Here's how the part is built. I have some questions about the finished solid (model axes, mm). Give positions to 0.01 mm unless a question says otherwise; leave off trailing zeros. Loops run counter-clockwise (first coordinate to the right, second up) from the corner with the lowest first, then second, coordinate; pieces in that order, holes last.
Q1. I'm going to push flat-ended pins straight in: P1, Ø4, axis at y = 23.5, z = 4, coming from the -X side; P2, Ø2.5, axis at y = 22.5, z = 3.5, coming from the +X side; P3, Ø5, axis at x = 93, y = -5, coming from the -Z side; P4, Ø4, axis at x = -65.5, z = 5.5, coming from the +Y side. Where does each tip first touch, or does it pass through?
Q2. Suppose I cut it at A-A (y = -19.5). List the corners of the cut face in (x, z) for me.
Q3. I need wall thicknesses on probe 1 along Y at (x, z) = (-71, 4.5); probe 2 along X at (y, z) = (16.5, 6.75). Which ranges of each line are inside material? Lowest first, please.
Q4. Suppose I cut it at B-B (x = -63). List the corners of the cut face in (y, z) for me.
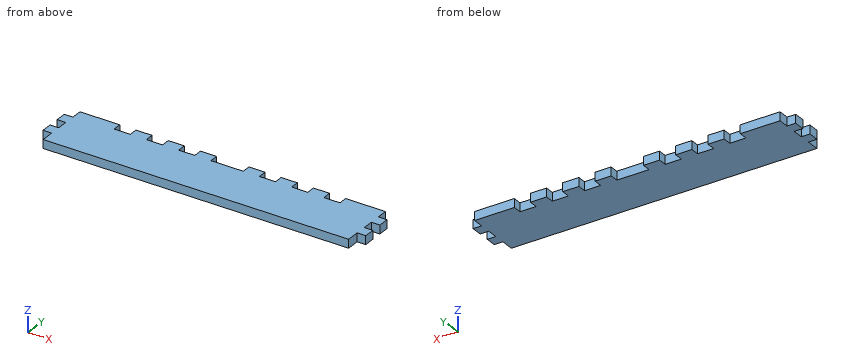
```python
from build123d import *

# Parameters (mm, degrees)
ESQUISSE1_W             = 300
ESQUISSE1_H             = 52
BOSS_EXTRU_1_DEPTH      = 8
ESQUISSE2_W             = 8
ESQUISSE2_H             = 10
ENL_V_MAT_EXTRU_1_DEPTH = 153.446712001
ESQUISSE3_W             = 8
ESQUISSE3_H             = 2
ENL_V_MAT_EXTRU_2_DEPTH = 153.446712001
ESQUISSE4_W             = 15
ESQUISSE4_H             = 8
ENL_V_MAT_EXTRU_3_DEPTH = 10


with BuildPart() as part:
    # Esquisse1 → Boss.-Extru.1 (new body)
    with BuildSketch(Plane.XY):
        Rectangle(ESQUISSE1_W, ESQUISSE1_H)
    extrude(amount=BOSS_EXTRU_1_DEPTH)

    # Esquisse2 → Enlèv. mat.-Extru.1 (cut, through all)
    with BuildSketch(Plane.XY):
        with Locations((-146, 1)):
            Rectangle(ESQUISSE2_W, ESQUISSE2_H)
        with Locations((-146, 21)):
            Rectangle(ESQUISSE2_W, ESQUISSE2_H)
        with Locations((-146, -19)):
            Rectangle(ESQUISSE2_W, ESQUISSE2_H)
    enl_v_mat_extru_1 = extrude(amount=ENL_V_MAT_EXTRU_1_DEPTH, mode=Mode.SUBTRACT)

    # Esquisse3 → Enlèv. mat.-Extru.2 (cut, through all)
    with BuildSketch(Plane.XY):
        with Locations((-146, -25)):
            Rectangle(ESQUISSE3_W, ESQUISSE3_H)
    enl_v_mat_extru_2 = extrude(amount=ENL_V_MAT_EXTRU_2_DEPTH, mode=Mode.SUBTRACT)

    # Symétrie1: Enlèv. mat.-Extru.1, Enlèv. mat.-Extru.2 across plane
    add(enl_v_mat_extru_1.mirror(Plane(origin=(0, 0, 0), x_dir=(0, 0, 1), z_dir=(1, 0, 0))), mode=Mode.SUBTRACT)
    add(enl_v_mat_extru_2.mirror(Plane(origin=(0, 0, 0), x_dir=(0, 0, 1), z_dir=(1, 0, 0))), mode=Mode.SUBTRACT)

    # Esquisse4 → Enlèv. mat.-Extru.3 (cut)
    with BuildSketch(Plane.XY):
        with Locations((-97.5, 22)):
            Rectangle(ESQUISSE4_W, ESQUISSE4_H)
        with Locations((-37.5, 22)):
            Rectangle(ESQUISSE4_W, ESQUISSE4_H)
        with Locations((37.5, 22)):
            Rectangle(ESQUISSE4_W, ESQUISSE4_H)
        with Locations((67.5, 22)):
            Rectangle(ESQUISSE4_W, ESQUISSE4_H)
        with Locations((97.5, 22)):
            Rectangle(ESQUISSE4_W, ESQUISSE4_H)
        with Locations((-67.5, 22)):
            Rectangle(ESQUISSE4_W, ESQUISSE4_H)
        Polygon((0, 18), (15, 18), (15, 26), (0, 26), (-15, 26), (-15, 18), align=None)
    extrude(amount=ENL_V_MAT_EXTRU_3_DEPTH, mode=Mode.SUBTRACT)


solid = part.part
```
Solutions:
1. P1: stops at x = -142
1. P2: stops at x = 142
1. P3: stops at z = 0
1. P4: stops at y = 18
2. outline: (-142, 0) - (142, 0) - (142, 8) - (-142, 8) - close
3. probe 1: y = -26 to 18
3. probe 2: x = -142 to 142
4. outline: (-26, 0) - (18, 0) - (18, 8) - (-26, 8) - close
